```python
from build123d import *

# Parameters (mm, degrees)
F0_W     = 57.15
F0_H     = 38.1
F1_DEPTH = 38.1
F3_DEPTH = 38.1
F5_DEPTH = 12.7
F9_DEPTH = 12.7


# Not quite as in the source:
# - a feature of the source that left no trace in its solid (it failed there, or was rolled back) is left out
# - a feature names something its author has since deleted; it is built from what else it names


with BuildPart() as f1:
    # F0 (on Front) → F1 (new body)
    with BuildSketch(Plane.XZ):
        with Locations((28.575, 19.05)):
            Rectangle(F0_W, F0_H)
    extrude(amount=F1_DEPTH)

    # F2 (on face) → F3 (cut)
    with BuildSketch(Plane.XZ.offset(38.1)):
        Polygon((57.15, 38.1), (44.45, 38.1), (57.15, 0), align=None)
    extrude(amount=-F3_DEPTH, mode=Mode.SUBTRACT)

    # F4 (on Front) → F5 (cut)
    with BuildSketch(Plane.XZ):
        Polygon((44.4645239406, 38.2572661593), (19.05, 38.2047749953), (31.75, 0), (57.1819730103, 0), align=None)
    extrude(amount=F5_DEPTH, mode=Mode.SUBTRACT)

    # F7 (on face) → F9 (cut)
    with BuildSketch(Plane.XZ.offset(38.1)):
        Polygon((44.45, 38.1), (14.2616005614, 38.1), (42.3013567924, 0), (57.15, 0), align=None)
    extrude(amount=-F9_DEPTH, mode=Mode.SUBTRACT)


solid = f1.part
```
Part model, mm, in its own coordinate system. A direction names the side the tool comes from. Round coordinates to 2 decimals unless told otherwise and drop trailing zeros. Write each loop counter-clockwise with the first axis right and the second up, starting at its lowest first coordinate (ties: lowest second). Pieces come first, ordered by that corner, then holes.
Item 1: Drop flat-ended pins along their axis: pin 1 Ø1 at (x, z) = (48.5, 14) entering from -Y; pin 2 Ø12 at (x, z) = (35, 12.5) entering from +Y; pin 3 Ø1.5 at (y, z) = (-12.5, 29.5) entering from +X. Give the stop position or say it passes through.
Results:
pin 1: stops at y = -25.4
pin 2: stops at y = -12.7
pin 3: stops at x = 47.56
Item 2: Cut at B-B, the plane x = 21. Give the cut face in (y, z).
Results:
outline: (-38.1, 0) - (0, 0) - (0, 32.34) - (-12.7, 32.34) - (-12.7, 38.1) - (-25.4, 38.1) - (-25.4, 28.94) - (-38.1, 28.94) - close
Item 3: Cut at C-C, the plane y = -24. Give the cut face in (x, z).
Results:
outline: (0, 0) - (57.15, 0) - (44.45, 38.1) - (0, 38.1) - close
Item 4: Cut at A-A, the plane z = 8.5. Give the cut face in (x, y).
Results:
outline: (0, -38.1) - (36.05, -38.1) - (36.05, -25.4) - (54.32, -25.4) - (54.32, -12.7) - (28.92, -12.7) - (28.92, 0) - (0, 0) - close
Item 5: Cut at D-D, the plane x = 41. Give the cut face in (y, z), plus the area to 3 significant figures.
Results:
outline: (-38.1, 0) - (-12.7, 0) - (-12.7, 38.1) - (-25.4, 38.1) - (-25.4, 1.77) - (-38.1, 1.77) - close
area: 506 mm2
Item 6: Which spindle directions (+Z, -Z, +X, -X, +Y, -Y) get a long thin tool onto all of the face, cutting with end or side? Do faces 1 (the flat face through (17, -19, 38.1)), 2 (the flat face through (40, -25.4, 24)), 3 (the flat face through (38, -12.7, 19)). Say none if no direction does.
Results:
face 1: +Z, +X, -X, +Y, -Y
face 2: +Z, +X, -Y
face 3: +Z, +X, +Y
Item 7: Probe L1, parallel to Y at x = 40.5, z = 28; L2, parallel to Y at x = 34, z = 5; L3, parallel to X at y = -10, z = 5.5. List the from-to ranges inside material, lowest first.
Results:
L1: y = -25.4 to -12.7
L2: y = -38.1 to -12.7
L3: x = 0 to 29.92
